Could you check a few things on this drawing? It's one solid part, dimensions in mm from its lowest x, y, z. Give positions to 0.01 mm unless a question says otherwise; leave off trailing zeros. Order: outer loops, then holes, each group sorted by start corner. A loop starts at its lowest first (then second) coordinate and runs counter-clockwise, first axis right, second up.
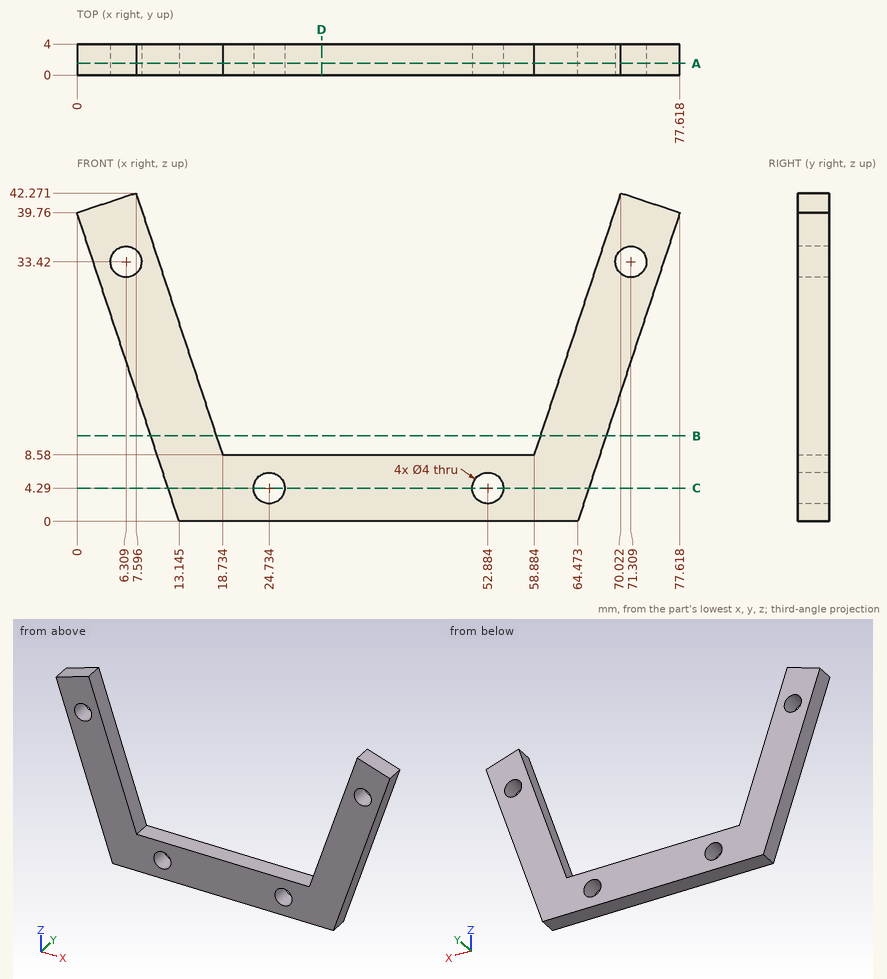
1) If I drill on line 1 (X direction, y = 1, z = 32) (1 decimal); line 2 (X direction, y = 2.5, z = 4.29) (1 decimal); line 3 (Z direction, x = 21, y = 3.6), over which ranges is the centre line in solid material (lowest first)?
2) Suppose I cut it at A-A (y = 1.5). Please give me the cut outline in (x, z) (1 decimal), and give its area (3 significant figures).
3) Suppose I cut it at D-D (x = 31.5). Please give me the cut outline in (y, z), and give its area (3 significant figures).
4) I'm going to push a flat-ended pin straight in: pin 1 Ø2 at (x, y) = (32, 2) entering from +Z. Where does the tip first touch, or does it pass through?
5) Suppose I cut it at C-C (z = 4.29). Please give me the cut outline in (x, y), and give its area (3 significant figures).
6) Suppose I cut it at B-B (z = 11). Please give me the cut outline in (x, y), and give its area (3 significant figures).
Results:
1. line 1: x = 2.6 to 4.9, 7.7 to 11, 66.6 to 69.9, 72.7 to 75.1
1. line 2: x = 11.7 to 22.7, 26.7 to 50.9, 54.9 to 65.9
1. line 3: z = 0 to 8.58
2. outline: (0, 39.8) - (13.1, 0) - (64.5, 0) - (77.6, 39.8) - (70, 42.3) - (58.9, 8.6) - (18.7, 8.6) - (7.6, 42.3) - close; hole circle Ø4 at (6.3, 33.4); hole circle Ø4 at (24.7, 4.3); hole circle Ø4 at (52.9, 4.3); hole circle Ø4 at (71.3, 33.4)
2. area: 961 mm2
3. outline: (0, 0) - (4, 0) - (4, 8.58) - (0, 8.58) - close
3. area: 34.3 mm2
4. pin 1: stops at z = 8.58
5. outline: (11.73, 0) - (22.73, 0) - (22.73, 4) - (11.73, 4) - close; (26.73, 0) - (50.88, 0) - (50.88, 4) - (26.73, 4) - close; (54.88, 0) - (65.89, 0) - (65.89, 4) - (54.88, 4) - close
5. area: 185 mm2
6. outline: (9.51, 0) - (17.93, 0) - (17.93, 4) - (9.51, 4) - close; (59.68, 0) - (68.11, 0) - (68.11, 4) - (59.68, 4) - close
6. area: 67.4 mm2
